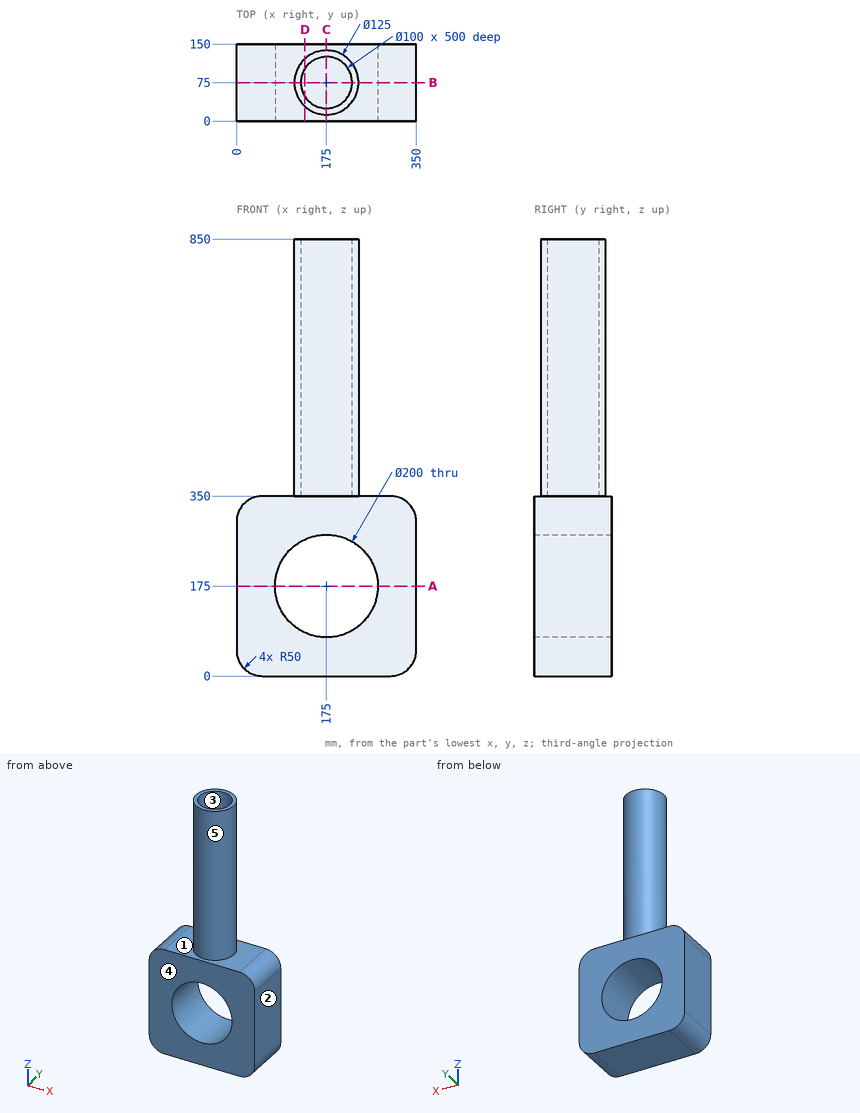
Geometry: see drawing. Coordinates: mm, zero at the bounding-box minimum. A direction names the side the tool comes from. Round coordinates to 2 decimals unless told otherwise and drop trailing zeros. Write each loop counter-clockwise with the first axis right and the second up, starting at its lowest first coordinate (ties: lowest second). Pieces come first, ordered by that corner, then holes.
Item 1: Mould query, pull axis X, two halves, no side actions, for the marked faces 1, 2 and 3. Classes: +X half, -X half, draft (parallel to the pull), parting line (faces both ways), or undercut.
Item 2: Section query A-A (z = 175). Return loops of the section in (x, y).
Item 3: Pin query (flat end, axial travel): P1, Ø5, axis at x = 161.5, y = 21.5, coming from the -Z side; P2, Ø1, axis at x = 51, y = 71.5, coming from the +Z side; P3, Ø10, axis at x = 310.5, y = 131.5, coming from the -Z side. Return the tip coordinate at first contact, or that it passes through.
Item 4: Section query B-B (y = 75). Return loops of the section in (x, z), plus the area to 3 significant figures.
Item 5: Section query D-D (x = 133). Return loops of the section in (y, z).
Item 6: Material intervals for L1, parallel to Y at x = 175, z = 739; L2, parallel to X at y = 65, z = 175; L3, parallel to Z at x = 283.5, y = 113.5, sorted ascending.
Item 7: Set-up query: the marked faces 4 and 5. Return all of +Z, -Z, +X, -X, +Y, -Y with unobstructed straight access to the full face (end or side cutting, diameter ignored); none if empty.
Item 8: Section query C-C (x = 175). Return loops of the section in (y, z), plus the area to 3 significant figures.
Completed:
1. face 1: draft
1. face 2: +X half
1. face 3: undercut
2. outline: (0, 0) - (75, 0) - (75, 150) - (0, 150) - close; (275, 0) - (350, 0) - (350, 150) - (275, 150) - close
3. P1: stops at z = 0
3. P2: stops at z = 350
3. P3: stops at z = 0.3
4. outline: (0, 50) arc R50 ccw to (50, 0) - (300, 0) arc R50 ccw to (350, 50) - (350, 300) arc R50 ccw to (300, 350) - (237.5, 350) - (237.5, 850) - (225, 850) - (225, 350) - (125, 350) - (125, 850) - (112.5, 850) - (112.5, 350) - (50, 350) arc R50 ccw to (0, 300) - close; hole circle Ø200 at (175, 175)
4. area: 101,000 mm2
5. outline: (0, 0) - (150, 0) - (150, 84.25) - (0, 84.25) - close; (0, 265.75) - (150, 265.75) - (150, 350) - (121.28, 350) - (121.28, 850) - (102.13, 850) - (102.13, 350) - (47.87, 350) - (47.87, 850) - (28.72, 850) - (28.72, 350) - (0, 350) - close
6. L1: y = 12.5 to 25, 125 to 137.5
6. L2: x = 0 to 75, 275 to 350
6. L3: z = 0 to 350
7. face 4: +Z, -Z, +X, -X, -Y
7. face 5: +Z
8. outline: (0, 0) - (150, 0) - (150, 75) - (0, 75) - close; (0, 275) - (150, 275) - (150, 350) - (137.5, 350) - (137.5, 850) - (125, 850) - (125, 350) - (25, 350) - (25, 850) - (12.5, 850) - (12.5, 350) - (0, 350) - close
8. area: 35,000 mm2
